```python
from build123d import *

# Parameters (mm, degrees)
F0_W   = 1.3
F0_H   = 2.5
F0_W_2 = 1.7
F0_W_3 = 2.5
F0_H_2 = 10.6689085803
F0_H_3 = 3.8655457098
F0_H_4 = 4
F0_H_5 = 16
F0_W_4 = 13.5


with BuildPart() as f1:
    # F0 (on Front) → F1 (revolve)
    with BuildSketch(Plane.XZ):
        with Locations((16.65, 14.8844542902)):
            Rectangle(F0_W, F0_H)
        Polygon((16, 13.6344542902), (16, 16.1344542902), (2.5, 16.1344542902), (2.5, 13.1048886105), align=None)
        with Locations((18.15, 14.8844542902)):
            Rectangle(F0_W_2, F0_H)
        with BuildLine():
            Line((2.5, 13.1048886105), (2.5, 16.1344542902))
            ThreePointArc((2.5, 16.1344542902), (1.767766953, 14.3666873372), (0, 13.6344542902))
            Line((0, 13.6344542902), (0, 11.1344542902))
            Line((0, 11.1344542902), (0, 10.6689085803))
            Line((0, 10.6689085803), (2.5, 10.6689085803))
            Line((2.5, 10.6689085803), (2.5, 13.1048886105))
        make_face()
        with Locations((18.15, 12.3844542902)):
            Rectangle(F0_W_2, F0_H)
        with BuildLine():
            Line((21.5, 13.6344542902), (19, 13.6344542902))
            Line((19, 13.6344542902), (19, 11.1344542902))
            Line((19, 11.1344542902), (21.5, 11.1344542902))
            ThreePointArc((21.5, 11.1344542902), (21.8535533906, 11.2809008996), (22, 11.6344542902))
            Line((22, 11.6344542902), (22, 13.1344542902))
            ThreePointArc((22, 13.1344542902), (21.8535533906, 13.4880076808), (21.5, 13.6344542902))
        make_face()
        Polygon((19, 11.1344542902), (17.3, 11.1344542902), (17.3, 10.6689085803), (17.3, 6.6344542902), (17.3, 4.0344542902), (17.3, 0), (17.3, -3.8655457098), (19, -3.8655457098), align=None)
        with Locations((1.25, 5.3344542902)):
            Rectangle(F0_W_3, F0_H_2)
        with Locations((1.25, -1.9327728549)):
            Rectangle(F0_W_3, F0_H_3)
        with BuildLine():
            Line((21.5, -3.8655457098), (19, -3.8655457098))
            Line((19, -3.8655457098), (19, -7.8655457098))
            Line((19, -7.8655457098), (21.5, -7.8655457098))
            ThreePointArc((21.5, -7.8655457098), (21.8535533906, -7.7190991004), (22, -7.3655457098))
            Line((22, -7.3655457098), (22, -4.3655457098))
            ThreePointArc((22, -4.3655457098), (21.8535533906, -4.0119923192), (21.5, -3.8655457098))
        make_face()
        with Locations((18.15, -5.8655457098)):
            Rectangle(F0_W_2, F0_H_4)
        with Locations((1.25, -5.8655457098)):
            Rectangle(F0_W_3, F0_H_4)
        with Locations((18.15, -15.8655457098)):
            Rectangle(F0_W_2, F0_H_5)
        with Locations((9.25, -15.8655457098)):
            Rectangle(F0_W_4, F0_H_5)
        with Locations((1.25, -15.8655457098)):
            Rectangle(F0_W_3, F0_H_5)
        with Locations((16.65, -15.8655457098)):
            Rectangle(F0_W, F0_H_5)
    revolve(axis=Axis((0, 0, -3.389431617), (0, 0, -1)))


solid = f1.part
```
Input: part model. Units: mm. Frame: model coordinates. A direction names the side the tool comes from. Round coordinates to 2 decimals unless told otherwise and drop trailing zeros. Write each loop counter-clockwise with the first axis right and the second up, starting at its lowest first coordinate (ties: lowest second). Pieces come first, ordered by that corner, then holes. Notation, with made-up numbers: (-14, 3.5) -> (23, 3.5) arc R28 ccw to (23, 27.5) -> close; hole circle Ø9 at (-32.5, 7.5). An arc over 180 degrees is marked (long way). Answer as CSV lines item,"result".
1. Ray query, L1, parallel to Y at x = 0, z = -2.25; L2, parallel to Z at x = 18.5, y = 8.5; L3, parallel to Z at x = 14, y = 9.5. Return the intervals inside material, ascending. Write a range as [from, to].
Geometry says:
L1,"y = [-19, -17.3], [-2.5, 2.5], [17.3, 19]"
L2,"z = [-7.87, -3.87], [11.13, 13.63]"
L3,"z = [-23.87, -7.87], [13.63, 16.13]"
2. Section B-B (x = 0). Give the number of separate pieces and of enclosed holes in the cut face, plus the area to 4 significant figures.
Geometry says:
separate pieces,"1"
enclosed holes,"2"
area,"919.5 mm^2"
3. Contact query for flat-ended pins moving along their axis: P1, Ø3, axis at y = 12, z = -9, coming from the +X side; P2, Ø8, axis at x = 8.5, z = -5.5, coming from the +Y side; P3, Ø4, axis at x = -12, z = -17, coming from the -Y side. Output: stop coordinate, or through.
Geometry says:
P1,"stops at x = 18.76"
P2,"stops at y = 21.53"
P3,"stops at y = -16.16"
4. Section C-C (z = -14.5). Return the cut outline in (x, y), plus the area to 3 significant figures.
Geometry says:
outline,"circle Ø38 at (0, 0)"
area,"1,130 mm^2"
5. Section A-A (z = 9). Return the cut outline in (x, y), plus the area to 3 significant figures.
Geometry says:
outline,"circle Ø38 at (0, 0); circle Ø5 at (0, 0); hole circle Ø34.6 at (0, 0)"
area,"214 mm^2"
6. Reachability of faces 5 (the flat face through (4, 0, -7.866)), 6 (the cylindrical face through (8.767, 16.856, 14.902)), 7 (the flat face through (-11, 16, -7.866)) from +Z, -Z, +X, -X, +Y, -Y: full face, straight path, thin tool, end or side. Return the list, or none.
Geometry says:
face 5,"none"
face 6,"+Z"
face 7,"-Z"
7. Mould query, pull axis X, two halves, no side actions, for faces 1 (the cylindrical face through (-0.54, 2.44, 2.77)), 2 (the flat face through (0, 4, 16.134)), 3 (the cylindrical face through (8.767, 16.856, -15.754)), 4 (the conical face through (-0.725, 3.265, 13.138)). Classes: +X half, -X half, draft (parallel to the pull), parting line (faces both ways), or undercut.
Geometry says:
face 1,"undercut"
face 2,"draft"
face 3,"parting line"
face 4,"undercut"
